Source: CAD feature listing. Evaluate the final solid. Frame: model axes, mm. A direction names the side the tool comes from. Give positions to 0.01 mm unless a question says otherwise; leave off trailing zeros. Order: outer loops, then holes, each group sorted by start corner. A loop starts at its lowest first (then second) coordinate and runs counter-clockwise, first axis right, second up.
```python
from build123d import *

# Parameters (mm, degrees)
SKETCH2_R               = 10.5
BOSS_EXTRUDE1_DEPTH     = 42
SKETCH3_R               = 12.5
BOSS_EXTRUDE2_DEPTH     = 4
SKETCH4_R               = 2.5
CUT_EXTRUDE1_DEPTH      = 12
CUT_EXTRUDE2_DEPTH      = 6
SKETCH6_R               = 12.5
SKETCH6_R_2             = 3.35
BOSS_EXTRUDE3_DEPTH     = 1
SKETCH8_W               = 3
SKETCH8_H               = 0.5
SKETCH8_W_2             = 0.5
SKETCH8_H_2             = 3
BOSS_EXTRUDE4_DEPTH     = 42
CHAMFER1_SIZE           = 1
CUT_EXTRUDE3_DEPTH      = 51.214539727
CUT_EXTRUDE3_DEPTH_BACK = 51.214539727
SKETCH7_R               = 3.5
BOSS_EXTRUDE11_DEPTH    = 10


with BuildPart() as part:
    # Sketch2 → Boss-Extrude1 (new body)
    with BuildSketch(Plane(origin=(0, 0, 0), x_dir=(1, 0, 0), z_dir=(0, 1, 0))):
        with Locations(Location((0, 0, 0), (0, 0, 90))):
            Circle(SKETCH2_R)
    extrude(amount=BOSS_EXTRUDE1_DEPTH)

    # Sketch3 → Boss-Extrude2 (add)
    with BuildSketch(Plane(origin=(0, 42, 0), x_dir=(1, 0, 0), z_dir=(0, 1, 0))):
        with Locations(Location((0, 0, 0), (0, 0, 270))):
            Circle(SKETCH3_R)
    extrude(amount=BOSS_EXTRUDE2_DEPTH)

    # Sketch4 → Cut-Extrude1 (cut)
    with BuildSketch(Plane(origin=(0, 46, 0), x_dir=(1, 0, 0), z_dir=(0, 1, 0))):
        with Locations(Location((0, 0, 0), (0, 0, 270))):
            Circle(SKETCH4_R)
    extrude(amount=-CUT_EXTRUDE1_DEPTH, mode=Mode.SUBTRACT)

    # Sketch5 → Cut-Extrude2 (cut)
    with BuildSketch(Plane.XZ.offset(-35)):
        Polygon((-4.734272207, 0), (-2.367136104, -4.1), (2.367136104, -4.1), (4.734272207, 0), (2.367136104, 4.1), (-2.367136104, 4.1), align=None)
    extrude(amount=-CUT_EXTRUDE2_DEPTH, mode=Mode.SUBTRACT)

    # Sketch6 → Boss-Extrude3 (add)
    with BuildSketch(Plane(origin=(0, 46, 0), x_dir=(1, 0, 0), z_dir=(0, 1, 0))):
        with Locations(Location((0, 0, 0), (0, 0, 270))):
            Circle(SKETCH6_R)
        with Locations(Location((0, 0, 0), (0, 0, 270))):
            Circle(SKETCH6_R_2, mode=Mode.SUBTRACT)
    extrude(amount=BOSS_EXTRUDE3_DEPTH)

    # Sketch8 → Boss-Extrude4 (add)
    with BuildSketch(Plane.XZ):
        Polygon((6.541030619, 8.662765176), (8.662350963, 6.541444833), (8.308797572, 6.187891442), (6.187477229, 8.309211786), align=None)
        with Locations((0, 10.5)):
            Rectangle(SKETCH8_W, SKETCH8_H)
        with Locations((10.501, 0.001)):
            Rectangle(SKETCH8_W_2, SKETCH8_H_2)
        Polygon((8.663765176, -6.540030619), (6.542444833, -8.661350963), (6.188891442, -8.307797572), (8.310211786, -6.186477229), align=None)
        with Locations((0.002, -10.5)):
            Rectangle(SKETCH8_W, SKETCH8_H)
        Polygon((-6.539030619, -8.662765176), (-8.660350963, -6.541444833), (-8.306797572, -6.187891442), (-6.185477229, -8.309211786), align=None)
        with Locations((-10.499, -0.001)):
            Rectangle(SKETCH8_W_2, SKETCH8_H_2)
        Polygon((-8.661765176, 6.540030619), (-6.540444833, 8.661350963), (-6.186891442, 8.307797572), (-8.308211786, 6.186477229), align=None)
    extrude(amount=-BOSS_EXTRUDE4_DEPTH)

    # Chamfer1
    chamfer1_edges = [part.edges().sort_by_distance(p)[0] for p in [
        (-4.016445773, 0, -9.70145161),
        (-1.498, 0, -10.571296662),
        (0.002, 0, -10.75),
        (1.502, 0, -10.571007987),
        (-9.700211661, 0, -4.019439479),
        (-8.534223693, 0, -6.415317563),
        (-7.599690791, 0, -7.602105005),
        (-6.412729118, 0, -8.536463676),
        (-9.700985019, 0, 4.017572607),
        (-10.570724567, 0, 1.499),
        (-10.749, 0, -0.001),
        (-10.570580229, 0, -1.501),
        (-4.01831274, 0, 9.700678467),
        (-6.414245443, 0, 8.535151573),
        (-7.601105005, 0, 7.600690791),
        (-8.535535893, 0, 6.413801336),
        (4.018039338, 0, 9.700791714),
        (1.5, 0, 10.571152423),
        (0, 0, 10.75),
        (-1.5, 0, 10.571152423),
        (9.700485123, 0, 4.018779463),
        (8.535651573, 0, 6.414745443),
        (7.601690791, 0, 7.602105005),
        (6.414301336, 0, 8.536035893),
        (9.701258362, 0, -4.01691252),
        (10.571724567, 0, -1.499),
        (10.751, 0, 0.001),
        (10.571580229, 0, 1.501),
        (4.019906186, 0, -9.700018261),
        (6.415817563, 0, -8.534723693),
        (7.603105005, 0, -7.600690791),
        (8.536963676, 0, -6.413229118),
    ]]
    chamfer(chamfer1_edges, length=CHAMFER1_SIZE)

    # Sketch7 → Cut-Extrude3 (cut, two sides: drawn at the far end of the back side and taken through both)
    with BuildSketch(Plane(origin=(0, 0, 0), x_dir=(0, 0, -1), z_dir=(1, 0, 0)).offset(-CUT_EXTRUDE3_DEPTH_BACK)):
        with Locations(Location((0, 17, 0), (0, 0, 64.604946599))):
            Circle(SKETCH7_R)
    extrude(amount=CUT_EXTRUDE3_DEPTH + CUT_EXTRUDE3_DEPTH_BACK, mode=Mode.SUBTRACT)


with BuildPart() as body_2:
    # Sketch36 → Boss-Extrude11 (new body)
    with BuildSketch(Plane(origin=(0, 0, 0), x_dir=(1, 0, 0), z_dir=(0, 1, 0))):
        with BuildLine():
            ThreePointArc((10.825317547, -6.25), (11.401622185, 5.123769272), (2.514051045, 12.244572158))
            ThreePointArc((2.514051045, 12.244572158), (1.821132072, 12.77615689), (1.810116753, 13.649425287))
            ThreePointArc((1.810116753, 13.649425287), (0, 16.5), (-1.810116753, 13.649425287))
            ThreePointArc((-1.810116753, 13.649425287), (-1.821132072, 12.77615689), (-2.514051045, 12.244572158))
            ThreePointArc((-2.514051045, 12.244572158), (-11.401622185, 5.123769272), (-10.825317547, -6.25))
            ThreePointArc((-10.825317547, -6.25), (-11.740381057, -9.665063509), (-15.155444566, -8.75))
            ThreePointArc((-15.155444566, -8.75), (-15.246255337, -7.69399267), (-14.493462435, -6.947868736))
            ThreePointArc((-14.493462435, -6.947868736), (-13.917395246, -6.415225062), (-13.903033251, -5.630778491))
            ThreePointArc((-13.903033251, -5.630778491), (-13.811642586, 5.851369845), (-5.626747062, 13.904665314))
            ThreePointArc((-5.626747062, 13.904665314), (-4.835213091, 14.484668262), (-4.41483231, 15.371352785))
            ThreePointArc((-4.41483231, 15.371352785), (0, 19), (4.41483231, 15.371352785))
            ThreePointArc((4.41483231, 15.371352785), (4.835213091, 14.484668262), (5.626747062, 13.904665314))
            ThreePointArc((5.626747062, 13.904665314), (13.811642586, 5.851369845), (13.903033251, -5.630778491))
            ThreePointArc((13.903033251, -5.630778491), (13.917395246, -6.415225062), (14.493462435, -6.947868736))
            ThreePointArc((14.493462435, -6.947868736), (15.246255337, -7.69399267), (15.155444566, -8.75))
            ThreePointArc((15.155444566, -8.75), (11.740381057, -9.665063509), (10.825317547, -6.25))
        make_face()
    extrude(amount=BOSS_EXTRUDE11_DEPTH)


solid = body_2.part
```
1) Section query C-C, the plane x = 0. Return the cut outline in (y, z), and give its area (3 significant figures).
Report:
outline: (0, -19) - (10, -19) - (10, -16.5) - (0, -16.5) - close
area: 25.0 mm2
2) Draft query along X for faces 3 (the cylindrical face through (-11.333, 4.93, -5.274)), 4 (the cylindrical face through (0, 5, -19)), 5 (the cylindrical face through (-4.844, 4.93, -14.474)), 6 (the cylindrical face through (4.826, 4.93, -14.495)). Return one class per face: +X half, -X half, draft (parallel to the pull), parting line (faces both ways), or undercut.
Report:
face 3: undercut
face 4: parting line
face 5: -X half
face 6: +X half
3) Section query D-D, the plane z = -3. Return the cut outline in (x, y).
Report:
outline: (-14.7, 0) - (-12.13, 0) - (-12.13, 10) - (-14.7, 10) - close; (12.13, 0) - (14.7, 0) - (14.7, 10) - (12.13, 10) - close
4) Reachability of faces 1 (the cylindrical face through (15.24, 4.93, 7.68)), 2 (the cylindrical face through (-1.816, 4.93, -12.788)) from +Z, -Z, +X, -X, +Y, -Y: full face, straight path, thin tool, end or side. Return the list, or none.
Report:
face 1: +X, +Y, -Y
face 2: +Y, -Y
5) Section query B-B, the plane y = 2.25. Return the cut outline in (x, z) (3 decimals), and give its area (3 significant figures).
Report:
outline: (-15.155, 8.75) arc R1.25 ccw to (-14.493, 6.948) arc R1 cw to (-13.903, 5.631) arc R15 ccw to (-5.627, -13.905) arc R2 cw to (-4.415, -15.371) arc R4.5 ccw to (4.415, -15.371) arc R2 cw to (5.627, -13.905) arc R15 ccw to (13.903, 5.631) arc R1 cw to (14.493, 6.948) arc R1.25 ccw to (15.155, 8.75) arc R2.5 ccw to (10.825, 6.25) arc R12.5 cw to (2.514, -12.245) arc R1 ccw to (1.81, -13.649) arc R2 cw (long way) to (-1.81, -13.649) arc R1 ccw to (-2.514, -12.245) arc R12.5 cw to (-10.825, 6.25) arc R2.5 ccw to start
area: 185 mm2
6) Section query A-A, the plane z = 7.5. Return the cut outline in (x, y), and give its area (3 significant figures).
Report:
outline: (-15.16, 0) - (-10.49, 0) - (-10.49, 10) - (-15.16, 10) - close; (10.49, 0) - (15.16, 0) - (15.16, 10) - (10.49, 10) - close
area: 93.3 mm2
7) Pin query (flat end, axial travel): pin 1 (3.5 mm diameter, centred on x = 0, z = -14.5, fed in from +Y); pin 2 (1.5 mm diameter, centred on y = 5, z = 2, fed in from +X); pin 3 (2 mm diameter, centred on x = 7, z = -13.5, fed in from -Y); pin 4 (6 mm diameter, centred on y = 1.5, z = 2.5, fed in from -X). Return the tip coordinate at first contact, or that it passes through.
Report:
pin 1: passes through
pin 2: stops at x = 14.95
pin 3: stops at y = 0
pin 4: stops at x = -15
8) Material intervals for L1, parallel to X at y = 8.25, z = 0.25; L2, parallel to X at y = 1, z = 3; L3, parallel to Z at x = 0, y = 6.75, sorted ascending.
Report:
L1: x = -15 to -12.5, 12.5 to 15
L2: x = -14.7 to -12.13, 12.13 to 14.7
L3: z = -19 to -16.5
